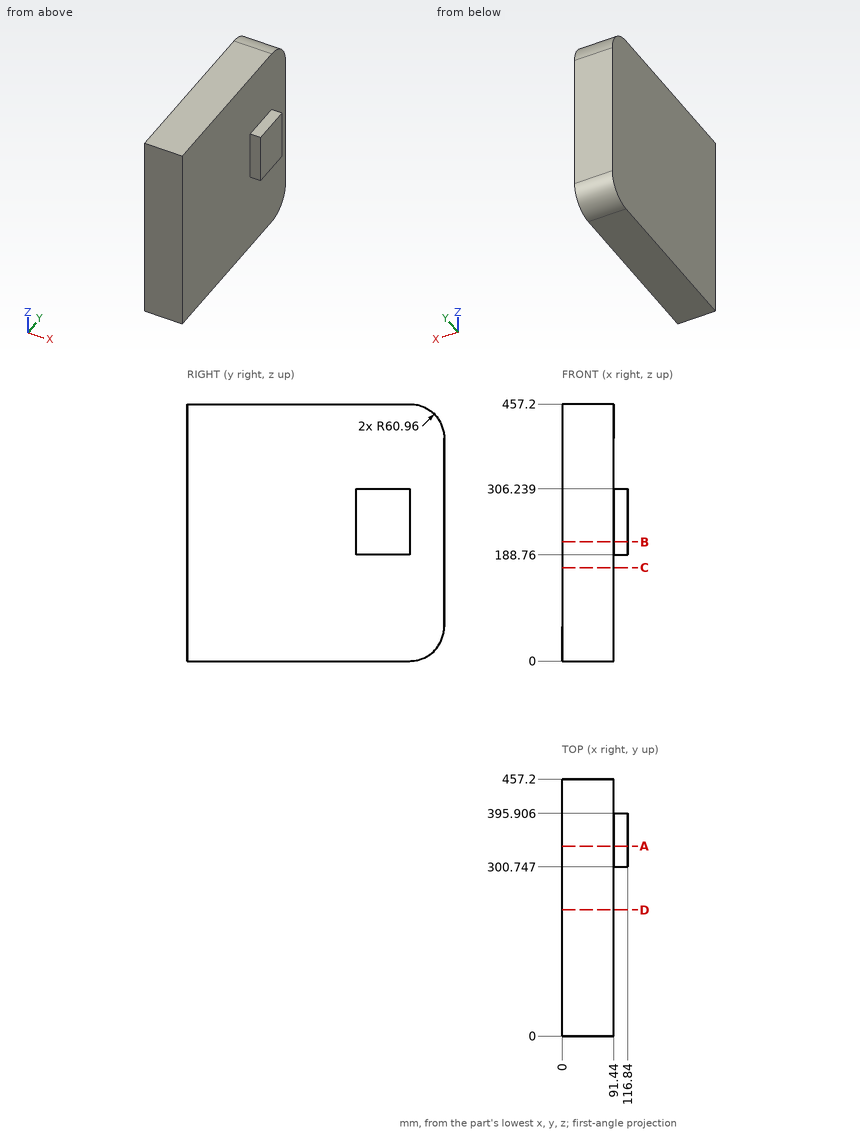
Input: dimensioned drawing with shaded views. Units: mm. Origin: part minimum x, y, z. Coordinates: 2 decimals unless noted, no trailing zeros. Order: outer loops, then holes, each group sorted by start corner. A loop starts at its lowest first (then second) coordinate and runs counter-clockwise, first axis right, second up.
(1) Material intervals for probe 1 along X at (y, z) = (275.5, 285.5); probe 2 along Z at (x, y) = (102.5, 305.5); probe 3 along Z at (x, y) = (29, 412), sorted ascending.
(2) Section query A-A (y = 338). Return the cut outline in (x, z), plus the area to 3 significant figures.
(3) Section query B-B (z = 212). Return the cut outline in (x, y) (1 decimal).
(4) First-contact query: pin 1 (5 mm diameter, centred on y = 204.5, z = 225.5, fed in from -X); pin 2 (1 mm diameter, centred on x = 96, z = 232.5, fed in from +Y) (1 decimal); pin 3 (2 mm diameter, centred on y = 351.5, z = 312.5, fed in from +X); pin 4 (20.5 mm diameter, centred on x = 103.5, z = 235.5, fed in from -Y). Flat tips, straight axial feed; report the tip coordinate or a pass-through.
(5) Section query C-C (z = 166). Return the cut outline in (x, y), plus the area to 3 significant figures.
Solution:
1. probe 1: x = 0 to 91.44
1. probe 2: z = 188.76 to 306.24
1. probe 3: z = 2.07 to 455.13
2. outline: (0, 0) - (91.44, 0) - (91.44, 188.76) - (116.84, 188.76) - (116.84, 306.24) - (91.44, 306.24) - (91.44, 457.2) - (0, 457.2) - close
2. area: 44,800 mm2
3. outline: (0, 0) - (91.4, 0) - (91.4, 300.7) - (116.8, 300.7) - (116.8, 395.9) - (91.4, 395.9) - (91.4, 457.2) - (0, 457.2) - close
4. pin 1: stops at x = 0
4. pin 2: stops at y = 395.9
4. pin 3: stops at x = 91.44
4. pin 4: stops at y = 300.75
5. outline: (0, 0) - (91.44, 0) - (91.44, 457.2) - (0, 457.2) - close
5. area: 41,800 mm2
